Check sheet for the modelled part. Datum: model origin and axes. Units: mm. A direction names the side the tool comes from. Coordinates: 2 decimals unless noted, no trailing zeros. Loops run counter-clockwise (first coordinate to the right, second up) from the corner with the lowest first, then second, coordinate; pieces in that order, holes last. Notation, with made-up numbers: (-37.5, -26) - (-29.5, -26) arc R18 ccw to (-29.5, -21) - close; hole circle Ø3 at (79, 23). An arc over 180 degrees is marked (long way). Use a Markdown table: item, result. Add a question column.
1) Sectioned sample at C-C, the plane z = 135.5. Enter the section's corners in (x, y).
2) Go/stop test with flat-tipped pins: P1, Ø4, axis at x = 5.5, z = 33, coming from the +Y side; P2, Ø5, axis at y = 0.5, z = -16.5, coming from the +X side; P3, Ø3, axis at y = -5, z = 159, coming from the +X side. Record where each tip stops, or that it passes through.
3) Tool access check on faces 1 (the cylindrical face through (-0.867, -3.905, 258.927)), 2 (the cylindrical face through (-0.867, -3.905, -34.51)), 3 (the flat face through (0, 0, 289)). Record the directions out of +Z, -Z, +X, -X, +Y, -Y that give a thin tool (end or side, any length) a straight path to the whole face; none if there is none.
4) Thickness scan on line 1 (Z direction, x = -17, y = -2); line 2 (Y direction, x = 1.5, z = 102); line 3 (Y direction, x = 9, z = 68). Record the ranges inside material, lowest first.
5) Sectioned sample at D-D, the plane z = -22. Enter the section's corners in (x, y).
6) Sectioned sample at A-A, the plane y = 0. Enter the section's corners in (x, z), then the cut area to 3 significant figures.
from build123d import *

# Parameters (mm, degrees)
SKETCH1_R           = 20.94
SKETCH1_R_2         = 4
SKETCH1_R_3         = 3.95
BOSS_EXTRUDE1_DEPTH = 228
SKETCH1_3_R         = 4
BOSS_EXTRUDE2_DEPTH = 70
BOSS_EXTRUDE4_START = 289
SKETCH1_5_R         = 4
SKETCH1_5_R_2       = 3.95
BOSS_EXTRUDE4_DEPTH = 61


with BuildPart() as part:
    # Sketch1 → Boss-Extrude1 (new body)
    # profile 1 of 3: a face of its own
    with BuildSketch(Plane.XY):
        with Locations(Location((0, 0, 0), (0, 0, 180))):
            Circle(SKETCH1_R)
        Circle(SKETCH1_R_2, mode=Mode.SUBTRACT)
    # profile 2 of 3: a face of its own
    with BuildSketch(Plane.XY):
        Circle(SKETCH1_R_2)
        Circle(SKETCH1_R_3, mode=Mode.SUBTRACT)
    # profile 3 of 3: a face of its own
    with BuildSketch(Plane.XY):
        Circle(SKETCH1_R_3)
    extrude(amount=BOSS_EXTRUDE1_DEPTH)

    # Sketch1<3> → Boss-Extrude2 (add)
    with BuildSketch(Plane.XY):
        Circle(SKETCH1_3_R)
    extrude(amount=-BOSS_EXTRUDE2_DEPTH)

    # Sketch1<5> → Boss-Extrude4 (add)
    # profile 1 of 2: a face of its own
    with BuildSketch(Plane.XY.offset(BOSS_EXTRUDE4_START)):
        Circle(SKETCH1_5_R)
        Circle(SKETCH1_5_R_2, mode=Mode.SUBTRACT)
    # profile 2 of 2: a face of its own
    with BuildSketch(Plane.XY.offset(BOSS_EXTRUDE4_START)):
        Circle(SKETCH1_5_R_2)
    extrude(amount=-BOSS_EXTRUDE4_DEPTH)


solid = part.part
Solved:
| question | item | result |
|---|---|---|
| 1 | outline | circle Ø41.88 at (0, 0) |
| 2 | P1 | stops at y = 20.65 |
| 2 | P2 | stops at x = 4 |
| 2 | P3 | stops at x = 20.65 |
| 3 | face 1 | +Z |
| 3 | face 2 | -Z |
| 3 | face 3 | +Z, +X, -X, +Y, -Y |
| 4 | line 1 | z = 0 to 228 |
| 4 | line 2 | y = -20.89 to 20.89 |
| 4 | line 3 | y = -18.91 to 18.91 |
| 5 | outline | circle Ø8 at (0, 0) |
| 6 | outline | (-20.94, 0) - (-4, 0) - (-4, -70) - (4, -70) - (4, 0) - (20.94, 0) - (20.94, 228) - (4, 228) - (4, 289) - (-4, 289) - (-4, 228) - (-20.94, 228) - close |
| 6 | area | 10,600 mm2 |
